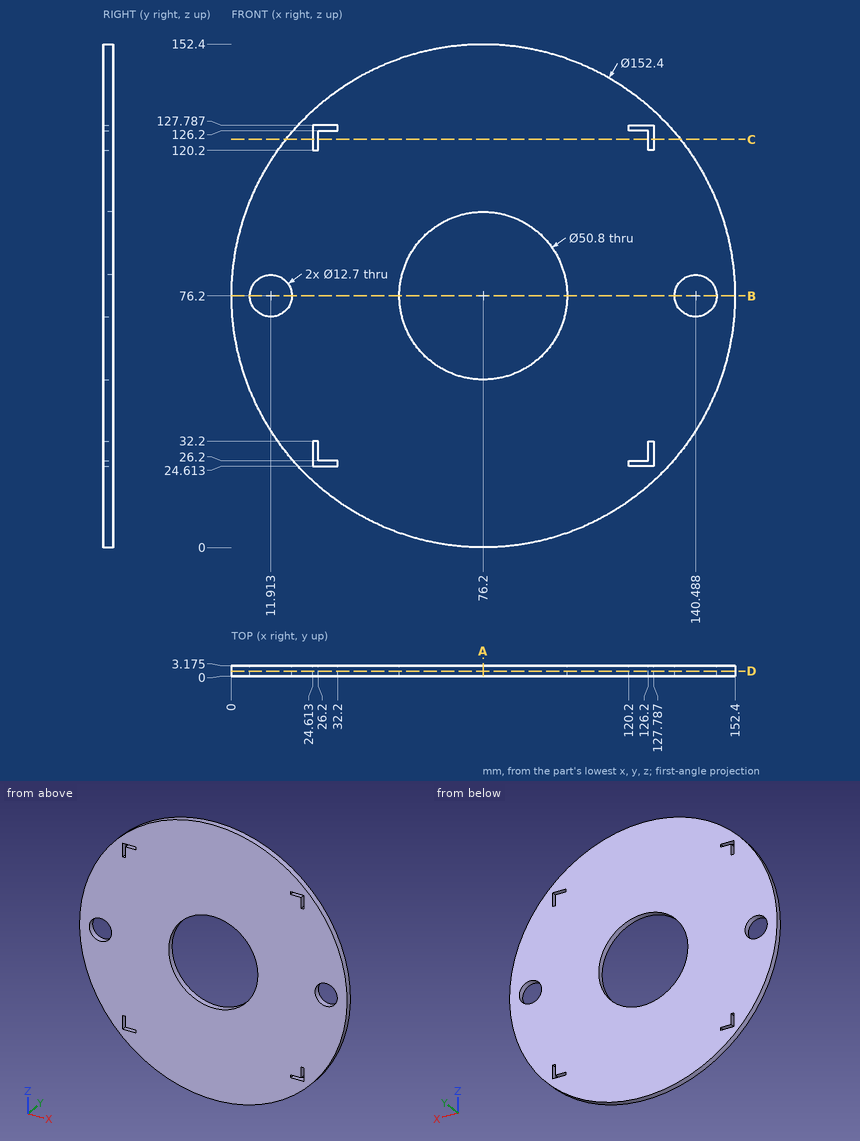
Answer from the drawing. Dimensions are ordinates in mm from the lowest x, y and z of the part. Coordinates: 2 decimals unless noted, no trailing zeros. Write each loop counter-clockwise with the first axis right and the second up, starting at its lowest first coordinate (ties: lowest second). Pieces come first, ordered by that corner, then holes. Notation, with made-up numbers: (20, 47) -> (46, 47) arc R35 ccw to (46, 84) -> close; hole circle Ø9 at (60.5, -25). An arc over 180 degrees is marked (long way). One line per question, with ' | ' between items.
1. Section C-C (z = 123.5) is taken. Determine the outline of the cut face in (x, y) (1 decimal).
Verdict:
outline: (16.5, 0) -> (24.6, 0) -> (24.6, 3.2) -> (16.5, 3.2) -> close; (26.2, 0) -> (126.2, 0) -> (126.2, 3.2) -> (26.2, 3.2) -> close; (127.8, 0) -> (135.9, 0) -> (135.9, 3.2) -> (127.8, 3.2) -> close
2. Straight lines are drawn through the part: line 1 (X direction, y = 1.35, z = 76.2); line 2 (Z direction, x = 143, y = 1.8) (1 decimal); line 3 (Z direction, x = 77.5, y = 1.6). For each, find the intervals that lie inside material, in ascending order.
Verdict:
line 1: x = 0 to 5.56, 18.26 to 50.8, 101.6 to 134.14, 146.84 to 152.4 | line 2: z = 39.5 to 70.4, 82 to 112.9 | line 3: z = 0.01 to 50.83, 101.57 to 152.39
3. Section B-B (z = 76.2) is taken. Determine the outline of the cut face in (x, y) (1 decimal).
Verdict:
outline: (0, 0) -> (5.6, 0) -> (5.6, 3.2) -> (0, 3.2) -> close; (18.3, 0) -> (50.8, 0) -> (50.8, 3.2) -> (18.3, 3.2) -> close; (101.6, 0) -> (134.1, 0) -> (134.1, 3.2) -> (101.6, 3.2) -> close; (146.8, 0) -> (152.4, 0) -> (152.4, 3.2) -> (146.8, 3.2) -> close
4. Section D-D (y = 1.5) is taken. Determine the outline of the cut face in (x, z).
Verdict:
outline: circle Ø152.4 at (76.2, 76.2); hole circle Ø12.7 at (11.91, 76.2); hole (24.61, 24.61) -> (32.2, 24.61) -> (32.2, 26.2) -> (26.2, 26.2) -> (26.2, 32.2) -> (24.61, 32.2) -> close; hole (24.61, 120.2) -> (26.2, 120.2) -> (26.2, 126.2) -> (32.2, 126.2) -> (32.2, 127.79) -> (24.61, 127.79) -> close; hole circle Ø50.8 at (76.2, 76.2); hole (120.2, 24.61) -> (127.79, 24.61) -> (127.79, 32.2) -> (126.2, 32.2) -> (126.2, 26.2) -> (120.2, 26.2) -> close; hole (120.2, 126.2) -> (126.2, 126.2) -> (126.2, 120.2) -> (127.79, 120.2) -> (127.79, 127.79) -> (120.2, 127.79) -> close; hole circle Ø12.7 at (140.49, 76.2)
5. Given pin 1 Ø0.5 at (x, y) = (127, 2) entering from +Z; pin 2 Ø1.7 at (x, y) = (25.5, 2) entering from +Z; pin 3 Ø1 at (x, y) = (123, 1) entering from +Z; pin 4 Ø2 at (x, z) = (84, 53.5) entering from +Y, each flat-ended and moving along its own axis, determine where each tip first touches the part or whether it passes through.
Verdict:
pin 1: stops at z = 133.22 | pin 2: stops at z = 133.83 | pin 3: stops at z = 136.72 | pin 4: passes through
6. Section A-A (x = 76.2) is taken. Determine the outline of the cut face in (y, z) (1 decimal).
Verdict:
outline: (0, 0) -> (3.2, 0) -> (3.2, 50.8) -> (0, 50.8) -> close; (0, 101.6) -> (3.2, 101.6) -> (3.2, 152.4) -> (0, 152.4) -> close
